Verification items for the finished model (mm, model axes). A direction names the side the tool comes from. Coordinates: 2 decimals unless noted, no trailing zeros. Order: outer loops, then holes, each group sorted by start corner. A loop starts at its lowest first (then second) coordinate and runs counter-clockwise, first axis right, second up. Notation, with made-up numbers: M -37.5,-34 L -15.5,-34 A25 cw -15.5,-9 Z; hole C 67,25.25 d8. An arc over 180 degrees is marked long. Answer as a JSON object with one key per item and string values. Group by question number.
(1) Gauge pin test, flat ends, axial feed: pin 1 Ø2 at (x, y) = (-11, 14.5) entering from +Z; pin 2 Ø6 at (x, y) = (-0.5, -17) entering from -Z; pin 3 Ø10 at (y, z) = (-13, 4) entering from -X. Record the tip position at first contact, or that the pin passes through.
(2) Cross-section at D-D (x = 12). Enter the section's corners in (y, z).
(3) Access from +Z, -Z, +X, -X, +Y, -Y to the whole of each face (thin tool, end or side, straight path). Record for faces 4 (the face through (0, 5, -2)), 5 (the face through (-0.69, -5.17, -23.27)), 6 (the face through (-14.211, 18, 16)).
(4) Material ranges on line 1 (Y direction, x = -12.25, z = -8); line 2 (Z direction, x = -5.25, y = -2); line 3 (Z direction, x = 5, y = 0), recorded low to high.
(5) Cross-section at A-A (z = 0). Enter the section's corners in (x, y), plus the area to 3 significant figures.
(6) Mould release check, pull along Y, two halves, no side actions. Record for faces 1 (the face through (15.668, -18, 16)), 2 (the face through (-6.5, -10.25, -2.28)), 3 (the face through (0.937, -6.514, -29.336)): released by +Y, released by -Y, zero draft, split by the parting line, or undercut.
(7) Cross-section at C-C (x = -9.5). Enter the section's corners in (y, z), plus the area to 3 significant figures.
from build123d import *

# Parameters (mm, degrees)
SKETCH2_R           = 10.500659562
SKETCH2_R_2         = 5
BOSS_EXTRUDE2_DEPTH = 13.182787508


with BuildPart() as part:
    # Sketch1 → Revolve1 (revolve)
    with BuildSketch(Plane.XY):
        with BuildLine():
            Line((10.667721535, 30.050515382), (15.667721535, 30.050515382))
            Line((15.667721535, 30.050515382), (15.667721535, 23.838456429))
            ThreePointArc((15.667721535, 23.838456429), (11.249332557, 12.133123747), (0, 6.656857557))
            Line((0, 6.656857557), (0, 10.500659562))
            ThreePointArc((0, 10.500659562), (9.779386002, 14.025882573), (13.211146798, 23.838456429))
            Line((13.211146798, 23.838456429), (-14.211146798, 23.838456429))
            Line((-14.211146798, 23.838456429), (-14.211146798, 30.050515382))
            Line((-14.211146798, 30.050515382), (-9.211146798, 30.050515382))
            Line((-9.211146798, 30.050515382), (10.667721535, 30.050515382))
        make_face()
    revolve(axis=Axis((0, 0, 0), (1, 0, 0)))

    # Sketch2 → Boss-Extrude2 (add)
    with BuildSketch(Plane.ZY):
        Circle(SKETCH2_R)
        Circle(SKETCH2_R_2, mode=Mode.SUBTRACT)
    extrude(amount=BOSS_EXTRUDE2_DEPTH)


solid = part.part
Taken from the geometry:
{
 "1": {"pin 1": "stops at z = 26.85", "pin 2": "stops at z = -26.59", "pin 3": "stops at x = -13.18"},
 "2": {"outline": "C 0,0 d60.1; C 0,0 d34.24; hole C 0,0 d47.68; hole C 0,0 d26.03"},
 "3": {"face 4": "+X", "face 5": "-X", "face 6": "+Z, -Z, -X, +Y, -Y"},
 "4": {"line 1": "y = -28.97 to -22.46, -6.8 to 6.8, 22.46 to 28.97", "line 2": "z = -29.98 to -23.75, -10.31 to -4.58, 4.58 to 10.31, 23.75 to 29.98", "line 3": "z = -30.05 to -23.84, -11.06 to -7.81, 7.81 to 11.06, 23.84 to 30.05"},
 "5": {"outline": "M -14.21,-30.05 L 15.67,-30.05 L 15.67,-23.84 A16.93 ccw 0,-6.66 L 0,-5 L -13.18,-5 L -13.18,-10.5 L 0,-10.5 A12.1 cw 13.21,-23.84 L -14.21,-23.84 Z; M -14.21,23.84 L 13.21,23.84 A12.1 cw 0,10.5 L -13.18,10.5 L -13.18,5 L 0,5 L 0,6.66 A16.93 ccw 15.67,23.84 L 15.67,30.05 L -14.21,30.05 Z", "area": "640 mm²"},
 "6": {"face 1": "zero draft", "face 2": "undercut", "face 3": "split by the parting line"},
 "7": {"outline": "C 0,0 d60.1; C 0,0 d21; hole C 0,0 d47.68; hole C 0,0 d10", "area": "1,320 mm²"}
}
